Verification items for the finished model (mm, model axes). A direction names the side the tool comes from. Round coordinates to 2 decimals unless told otherwise and drop trailing zeros. Order: outer loops, then holes, each group sorted by start corner. A loop starts at its lowest first (then second) coordinate and runs counter-clockwise, first axis right, second up. Notation, with made-up numbers: (77.5, -8.5) -> (82.5, -8.5) arc R31 ccw to (82.5, 16.5) -> close; hole circle Ø8 at (7, 79). An arc over 180 degrees is marked (long way). Return JSON: item names as keys, results as strings. Group by question number.
1) Section check C-C on x = 11.25. State how many separate pieces and enclosed holes the cut face has, plus the area to 3 significant figures.
2) Section check A-A on x = 17.75. Enter the section's corners in (y, z).
3) Depth check by flat-ended pin: pin 1 (2 mm diameter, centred on x = 11.5, z = -7, fed in from +Y); pin 2 (8 mm diameter, centred on x = 6.5, y = -10, fed in from +Z); pin 3 (1.5 mm diameter, centred on y = -3.5, z = 0.5, fed in from +X). Enter the tip coordinate at first touch or a pass-through.
4) Tool access check on faces 4 (the cylindrical face through (12.99, -4.26, 10.14)), 5 (the flat face through (12, 0, 0)), 6 (the flat face through (17.986, -1.227, -11.675)), 7 (the flat face through (17, -7.5, -7.5)). Record the directions out of +Z, -Z, +X, -X, +Y, -Y that give a thin tool (end or side, any length) a straight path to the whole face; none if there is none.
5) Draft check along Y on faces 1 (the flat face through (13, -12, 0)), 2 (the cylindrical face through (12.99, 10.14, 4.26)), 3 (the cylindrical face through (13.5, 7.3, -7.2)). Enter one of: pulls with the +Y half, pulls with the -Y half, needs draft (parallel to the pull), parting line crosses it, or undercut.
6) Scan lines: L1, parallel to X at y = -5.25, z = -10; L2, parallel to Y at x = 19.4, z = 0; L3, parallel to X at y = 1.75, z = -1.5. Record each from-to range of solid material in increasing order.
Autodesk Inventor part; units mm, degrees
ref_plane "YZ Plane" through (0, 0, 0) normal (1, 0, 0) x (0, 1, 0)
ref_plane "XZ Plane" through (0, 0, 0) normal (0, 1, 0) x (-1, 0, 0)
ref_plane "XY Plane" through (0, 0, 0) normal (0, 0, 1) x (1, 0, 0)
sketch "Sketch1" plane through (0, 0, 0) normal (1, 0, 0) x (0, 1, 0)
  circle A0 centre (0, 0) radius 12.5
  circle A1 centre (0, 0) radius 11
  dimension "d0" = 25
  dimension "d1" = 22
extrude "Extrusion1" add sketch "Sketch1" along normal blind 6.5
sketch "Sketch2" plane through (6.5, 0, 0) normal (1, 0, 0) x (0, 0, -1)
  circle A0 centre (0, 0) radius 9
  circle A1 centre (0, 0) radius 12.5
  dimension "d4" = 18
extrude "Extrusion2" add sketch "Sketch2" along normal blind 5.5
sketch "Sketch3" plane through (12, 0, 0) normal (1, 0, 0) x (0, 0, -1)
  circle A0 centre (0, 0) radius 11
  dimension "d55" = 22
extrude "Extrusion3" add sketch "Sketch3" along normal blind 2
sketch "Sketch4" plane through (14, 0, 0) normal (1, 0, 0) x (0, 0, -1)
  circle A0 centre (0, 0) radius 12.5
extrude "Extrusion4" add sketch "Sketch4" along normal blind 3
sketch "Sketch5" plane through (17, 0, 0) normal (1, 0, 0) x (0, 0, -1)
  circle A0 centre (0, 0) radius 9
  circle A1 centre (0, 0) radius 11
  dimension "d54" = 22
extrude "Extrusion5" add sketch "Sketch5" along normal blind 2
sketch "Sketch7" plane through (17, 0, 0) normal (1, 0, 0) x (0, 0, -1)
  line L0 (0, 0) -> (6.2, 0)
  line L1 (0, 0) -> (-3.1, 5.3694)
  line L2 (0, 0) -> (6.2, 0) construction
  line L3 (0, 0) -> (-3.1, -5.3694)
  line L4 (0, 0) -> (6.2, 0) construction
  dimension "d15" = 6.2
  dimension "d16" = 6.2
  dimension "d17" = 120
  dimension "d18" = 6.2
  dimension "d19" = 120
hole "Hole1" at (17, 5.3694, 3.1) at (17, 0, -6.2) at (17, -5.3694, 3.1) direction (-1, 0, 0) diameter 3.4 end through all
sketch "Sketch8" plane through (12, 0, 0) normal (1, 0, 0) x (0, 0, -1)
  circle A0 centre (0, 0) radius 9
  circle A1 centre (0, 0) radius 9
  circle A2 centre (0, 0) radius 12.5
  line L0 (-9, 0) -> (-12.5, 0)
  line L1 (-8.9507, 0.9408) -> (-12.4315, 1.3066)
  line L2 (-0.9408, -8.9507) -> (-1.3066, -12.4315)
  circle A3 centre (0, 0) radius 12.5
  line L3 (0, -12.5) -> (0, -9)
  line L4 (9, 0) -> (12.5, 0)
  line L5 (0.9408, 8.9507) -> (1.3066, 12.4315)
  line L6 (0, 12.5) -> (0, 9)
  line L7 (-0.2849, 0.0299) -> (8.8591, 0.0299) construction
  line L8 (8.9507, -0.9408) -> (12.4315, -1.3066)
extrude "Extrusion7" add sketch "Sketch8" along normal blind 7 contours L4 A2 L8 A0 | A0 L6 A2 L5 | L3 A2 L2 A0 | A0 L0 A2 L1
sketch "Sketch10" plane through (17, 0, 0) normal (1, 0, 0) x (0, 0, -1)
  circle A0 centre (0, 0) radius 11
  circle A1 centre (0, 11) radius 0.75
  arc A2 (-11, 0) -> (-1.1498, -10.9397) centre (0, 0) ccw
  circle A3 centre (-11, 0) radius 0.75
  line L0 (0, -11) -> (0, -12.5)
  circle A4 centre (0, -11) radius 0.75
  circle A5 centre (11, 0) radius 0.75
  line L1 (0, 0) -> (10.9982, 0) construction
  line L2 (0, 0) -> (7.7782, 7.7782)
  line L3 (0, 0) -> (11, 0) construction
  circle A6 centre (7.7782, 7.7782) radius 0.75
  line L4 (0, 0) -> (-7.7782, 7.7782)
  line L5 (0, 0) -> (-7.7782, -7.7782)
  line L6 (0, 0) -> (7.7782, -7.7782)
  circle A7 centre (-7.7782, -7.7782) radius 0.75
  circle A8 centre (7.7782, -7.7782) radius 0.75
  circle A9 centre (-7.7782, 7.7782) radius 0.75
  dimension "d60" = 1.5
  dimension "d61" = 1.5
  dimension "d62" = 1.5
  dimension "d63" = 1.5
  dimension "d66" = 11
  dimension "d67" = 45
  dimension "d68" = 1.5
  dimension "d69" = 11
  dimension "d70" = 11
  dimension "d71" = 11
  dimension "d72" = 1.5
  dimension "d73" = 1.5
  dimension "d74" = 1.5
extrude "Extrusion8" cut sketch "Sketch10" against normal blind 7 contours A0 A5 | A0 A5 | A6 L2 A0 | A0 A6 | A8 A0 | A0 L6 A8 | L2 A6 A0 | A0 A8 L6 | A1 A0 | A0 A1 | A9 A0 L4 | L4 A0 A9 | A7 A0 L5 | L5 A0 A7 | A0 A9 | A0 A7 | A3 A0 | A0 A3
sketch "Sketch11" plane through (19, 0, 0) normal (1, 0, 0) x (0, 0, -1)
  circle A0 centre (0, 0) radius 9
  circle A1 centre (0, 0) radius 12.5
  dimension "d77" = 18
  dimension "d78" = 25
extrude "Extrusion9" add sketch "Sketch11" along normal blind 4
properties part number "felga"
Check result:
{
 "1": {"separate pieces": "1", "enclosed holes": "8", "area": "224 mm^2"},
 "2": {"outline": "(-12.5, 0) -> (-11, 0) arc R11 ccw to (-1.15, -10.94) -> (-1.31, -12.43) arc R12.5 ccw to (0, -12.5) -> (0, -11) arc R11 ccw to (10.94, -1.15) -> (12.43, -1.31) arc R12.5 ccw to (12.5, 0) -> (11, 0) arc R11 ccw to (1.15, 10.94) -> (1.31, 12.43) arc R12.5 ccw to (0, 12.5) -> (0, 11) arc R11 ccw to (-10.94, 1.15) -> (-12.43, 1.31) arc R12.5 ccw to start; hole circle Ø18 at (0, 0)"},
 "3": {"pin 1": "y = 10.97", "pin 2": "z = 10.97", "pin 3": "x = 17"},
 "4": {"face 4": "+Z, -Y", "face 5": "-X", "face 6": "-Y", "face 7": "none"},
 "5": {"face 1": "needs draft", "face 2": "pulls with the +Y half", "face 3": "undercut"},
 "6": {"L1": "0 to 12, 14 to 17, 19 to 23", "L2": "-12.5 to -9, 9 to 12.5", "L3": "12 to 17"}
}
